from build123d import *

# Parameters (mm, degrees)
F0_W     = 38.1
F0_H     = 50.8
F1_DEPTH = 22.225
F3_DEPTH = 50.801
F4_SIZE  = 1


with BuildPart() as f1:
    # F0 (on Top) → F1 (new body)
    with BuildSketch(Plane.XY):
        with Locations((19.05, 25.4)):
            Rectangle(F0_W, F0_H)
    extrude(amount=F1_DEPTH)

    # F2 (on face) → F3 (cut, through all)
    with BuildSketch(Plane.XZ):
        Polygon((38.1, 15.875), (22.225, 0), (38.1, 0), align=None)
        Polygon((0, 0), (15.875, 0), (0, 15.875), align=None)
    extrude(amount=-F3_DEPTH, mode=Mode.SUBTRACT)

    # F4
    f4_edges = [f1.edges().sort_by_distance(p)[0] for p in [
        (30.1625, 0, 7.9375),
        (7.9375, 0, 7.9375),
        (30.1625, 50.8, 7.9375),
        (7.9375, 50.8, 7.9375),
    ]]
    chamfer(f4_edges, length=F4_SIZE)


solid = f1.part
Geometry: final body of the model. Coordinates: model frame, mm. Give positions to 0.01 mm unless a question says otherwise; leave off trailing zeros. Loops run counter-clockwise (first coordinate to the right, second up) from the corner with the lowest first, then second, coordinate; pieces in that order, holes last. Notation, with made-up numbers: (37, 25) - (63, 25) arc R14 ccw to (63, 30) - close; hole circle Ø11 at (83, -1.75). An arc over 180 degrees is marked (long way). One line per question, with ' | ' between items. Start each with the question number.
(1) Contact query for flat-ended pins moving along their axis: pin 1 (8 mm diameter, centred on y = 26, z = 6, fed in from -X) (3 decimals); pin 2 (12 mm diameter, centred on x = 4.5, y = 9.5, fed in from -Z) (3 decimals). Output: stop coordinate, or through.
(2) Ray query, line 1 (Z direction, x = 7.5, y = 19) (3 decimals); line 2 (Z direction, x = 30.5, y = 41) (3 decimals); line 3 (X direction, y = 24, z = 15.5) (3 decimals). Return the intervals inside material, ascending. Write a range as from..to.
(3) Section query B-B on y = 43. Return loops of the section in (x, z) (3 decimals), then the cut area to 3 significant figures.
(4) Section query C-C on x = 5. Return loops of the section in (y, z) (3 decimals).
(5) Section query A-A on z = 12. Return loops of the section in (x, y) (3 decimals).
(6) Section query D-D on z = 7. Return loops of the section in (x, y) (3 decimals), then the cut area to 3 significant figures.
The answers:
1) pin 1: x = 5.875 | pin 2: z = 5.375
2) line 1: 8.375..22.225 | line 2: 8.275..22.225 | line 3: 0.375..37.725
3) outline: (0, 15.875) - (15.875, 0) - (22.225, 0) - (38.1, 15.875) - (38.1, 22.225) - (0, 22.225) - close | area: 595 mm2
4) outline: (0, 12.289) - (1, 10.875) - (49.8, 10.875) - (50.8, 12.289) - (50.8, 22.225) - (0, 22.225) - close
5) outline: (3.875, 1) - (5.289, 0) - (32.811, 0) - (34.225, 1) - (34.225, 49.8) - (32.811, 50.8) - (5.289, 50.8) - (3.875, 49.8) - close
6) outline: (8.875, 1) - (10.289, 0) - (27.811, 0) - (29.225, 1) - (29.225, 49.8) - (27.811, 50.8) - (10.289, 50.8) - (8.875, 49.8) - close | area: 1,030 mm2
